The listing builds one solid part. Answer for the finished solid, in the listing's coordinates (mm). Face numbers are marked on the shaded views. A direction names the side the tool comes from. Coordinates: 2 decimals unless noted, no trailing zeros. Order: outer loops, then holes, each group sorted by start corner. A loop starts at its lowest first (then second) coordinate and runs counter-clockwise, first axis right, second up. Notation, with made-up numbers: (83, 88) -> (97, 88) arc R28 cw to (97, 125) -> close; hole circle Ø11 at (-8, 76.5). An arc over 180 degrees is marked (long way). Write each question's results on one line, items separated by ' | '. Start each with the question number.
(1) The part is cut by section B-B, the plane z = 19. Give the vertices of the cut face in (x, y).
(2) Given pin 1 (5 mm diameter, centred on x = -6.5, z = -8, fed in from -Y); pin 2 (1.3 mm diameter, centred on y = 0, z = 0.5, fed in from -X); pin 3 (6 mm diameter, centred on x = -1.5, z = -25, fed in from -Y); pin 4 (2 mm diameter, centred on y = 20, z = -15, fed in from -X), each flat-ended and moving along its own axis, determine where each tip first touches the part or whether it passes through.
(3) The part is cut by section C-C, the plane y = 7.5. Give the vertices of the cut face in (x, z).
(4) Determine the mould class of the marked faces 1, 2 and 3 for opening direction Z: +Z half, -Z half, draft (parallel to the pull), parting line (faces both ways), or undercut.
(5) Straight lines are drawn through the part: L1, parallel to Z at x = 16, y = 4.25; L2, parallel to Z at x = -6.5, y = 5.15; L3, parallel to Y at x = -7.5, z = 2. For each, find the intervals that lie inside material, in ascending order.
(6) A tool of negligible diameter and unlimited length cuts with its end or side. For the marked faces 4, 5 and 6, from which of +Z, -Z, +X, -X, +Y, -Y can it reach the whole face along a straight path? Write none if from no direction.
(7) The part is cut by section A-A, the plane z = -25. Give the vertices of the cut face in (x, y), then the cut area to 3 significant figures.
(8) The part is cut by section D-D, the plane y = 27. Give the vertices of the cut face in (x, z).
Autodesk Inventor part; units mm, degrees
ref_plane "YZ Plane" through (0, 0, 0) normal (1, 0, 0) x (0, 1, 0)
ref_plane "XZ Plane" through (0, 0, 0) normal (0, 1, 0) x (-1, 0, 0)
ref_plane "XY Plane" through (0, 0, 0) normal (0, 0, 1) x (1, 0, 0)
ref_plane "Work Plane5" through (0, 3, 0) normal (0, 1, 0) x (1, 0, 0)
sketch "Sketch45" plane through (0, 3, 0) normal (0, 1, 0) x (1, 0, 0)
  line L0 (35, -20) -> (-3, -20)
  line L1 (-3, -20) -> (-3, 20)
  line L2 (-3, 20) -> (35, 20)
  line L3 (35, 20) -> (35, -20)
  point P0 (0, 0)
  dimension "d142" = 38
  dimension "d143" = 40
extrude "Extrusion34" add sketch "Sketch45" along normal blind 30
ref_plane "Work Plane2" through (0, 0, 0) normal (0, -1, 0) x (1, 0, 0)
sketch "Sketch47" plane through (0, 0, 0) normal (0, -1, 0) x (1, 0, 0)
  circle A0 centre (16, 0) radius 18
  point P0 (0, 0)
  dimension "d146" = 36
extrude "Extrusion35" cut sketch "Sketch47" against normal blind 30 draft -15
ref_plane "Work Plane1" through (0, 3, 0) normal (0, 1, 0) x (1, 0, 0)
sketch "Sketch74" plane through (0, 33, 0) normal (0, 1, 0) x (1, 0, 0)
  circle A0 centre (20, 0) radius 1.15
  point P0 (0, 0)
  dimension "d210" = 2.3
extrude "Extrusion51" cut sketch "Sketch74" against normal blind 10
sketch "Sketch77" plane through (0, 3, 0) normal (0, -1, 0) x (1, 0, 0)
  circle A0 centre (16, 0) radius 17.5
  point P0 (0, 0)
  dimension "d219" = 35
sketch "Sketch78" plane through (0, 3, 0) normal (0, -1, 0) x (1, 0, 0)
  line L0 (45, -30) -> (-13, -30)
  line L1 (-13, -30) -> (-13, 30)
  line L2 (-13, 30) -> (45, 30)
  line L3 (45, 30) -> (45, -30)
  line L4 (45, -30) -> (-13, 30) construction
  line L5 (-13, -30) -> (45, 30) construction
  point P0 (0, 0)
  point P1 (16, 0)
  dimension "d220" = 58
  dimension "d221" = 60
extrude "Extrusion53" add sketch "Sketch78" against normal blind 3
extrude "Extrusion54" cut sketch "Sketch77" against normal blind 3
sketch "Sketch81" plane through (0, 3, 0) normal (0, -1, 0) x (1, 0, 0)
  circle A0 centre (33.5, -25) radius 2.7
  line L0 (-13, -30) -> (45, -30)
  line L1 (45, -30) -> (45, 30)
  circle A1 centre (16, -25) radius 2.7
  circle A2 centre (-1.5, -25) radius 2.7
  circle A3 centre (-6.5, -8) radius 2.7
  circle A4 centre (-6.5, 8) radius 2.7
  circle A5 centre (-1.5, 25) radius 2.7
  circle A6 centre (16, 25) radius 2.7
  circle A7 centre (33.5, 25) radius 2.7
  point P0 (0, 0)
  dimension "mag_D" = 5.4
  dimension "d232" = 5
  dimension "d233" = 11.5
  dimension "d234" = 5.4
  dimension "d235" = 17.5
  dimension "d236" = 5.4
  dimension "d237" = 17.5
  dimension "d238" = 5.4
  dimension "d239" = 5
  dimension "d240" = 17
  dimension "d241" = 5.4
  dimension "d242" = 16
  dimension "d243" = 5.4
  dimension "d244" = 17
  dimension "d245" = 5.4
  dimension "d246" = 17.5
  dimension "d247" = 5.4
  dimension "d248" = 17.5
  dimension "d249" = 5
extrude "Extrusion56" cut sketch "Sketch81" against normal blind 30
sketch "Sketch83" plane through (0, 3, 0) normal (0, -1, 0) x (1, 0, 0)
  circle A0 centre (-6.5, -8) radius 2.7
  line L0 (-9.1417, -2.4) -> (-9.1417, 2.4)
  line L1 (-9.1417, 2.4) -> (-4.9848, 0)
  line L2 (-4.9848, 0) -> (-9.1417, -2.4)
  point P0 (0, 0)
  point P1 (-9.1417, -8.5581)
  point P2 (-7.756, 0)
  dimension "d253" = 4.8
extrude "Extrusion57" add sketch "Sketch83" along normal blind 4.5 contours L0 L1 L2
equation "\"d234\" = mag_D"
equation "\"d236\" = mag_D"
equation "\"d237\" = d235"
equation "\"d238\" = mag_D"
equation "\"d241\" = mag_D"
equation "\"d243\" = mag_D"
equation "\"d244\" = d240"
equation "\"d245\" = mag_D"
equation "\"d246\" = d235"
equation "\"d247\" = mag_D"
equation "\"d248\" = d235"
equation "\"d249\" = d239"
properties part number "liquid_port_v03"
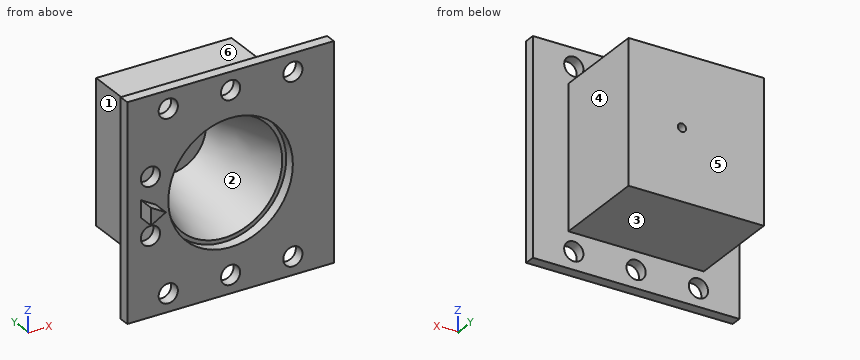
Established:
1) outline: (-13, 3) -> (45, 3) -> (45, 6) -> (35, 6) -> (35, 33) -> (-3, 33) -> (-3, 6) -> (-13, 6) -> close
2) pin 1: passes through | pin 2: stops at x = -9.14 | pin 3: stops at y = 3 | pin 4: stops at x = -3
3) outline: (-3, -20) -> (35, -20) -> (35, 20) -> (-3, 20) -> close; hole circle Ø31.98 at (16, 0)
4) face 1: draft | face 2: undercut | face 3: -Z half
5) L1: z = -30 to -27.7, -22.3 to -17.5, 17.5 to 22.3, 27.7 to 30 | L2: z = -30 to -10.7, -5.3 to 5.3, 10.7 to 30 | L3: y = 3 to 6
6) face 4: +Z, -Z, +X, +Y | face 5: +Z, -Z, +X, -X, +Y | face 6: +Z, +X, -X, +Y
7) outline: (-13, 3) -> (-4.2, 3) -> (-4.2, 6) -> (-13, 6) -> close; (1.2, 3) -> (13.3, 3) -> (13.3, 6) -> (1.2, 6) -> close; (18.7, 3) -> (30.8, 3) -> (30.8, 6) -> (18.7, 6) -> close; (36.2, 3) -> (45, 3) -> (45, 6) -> (36.2, 6) -> close | area: 125 mm^2
8) outline: (-3, -20) -> (35, -20) -> (35, 20) -> (-3, 20) -> close; hole circle Ø21.53 at (16, 0)
